Design review of the part shown in the three views and the two pictorial views. Dimensions are in mm from the part's minimum x, y and z. Round coordinates to 2 decimals unless told otherwise and drop trailing zeros. Order: outer loops, then holes, each group sorted by start corner. A loop starts at its lowest first (then second) coordinate and runs counter-clockwise, first axis right, second up.
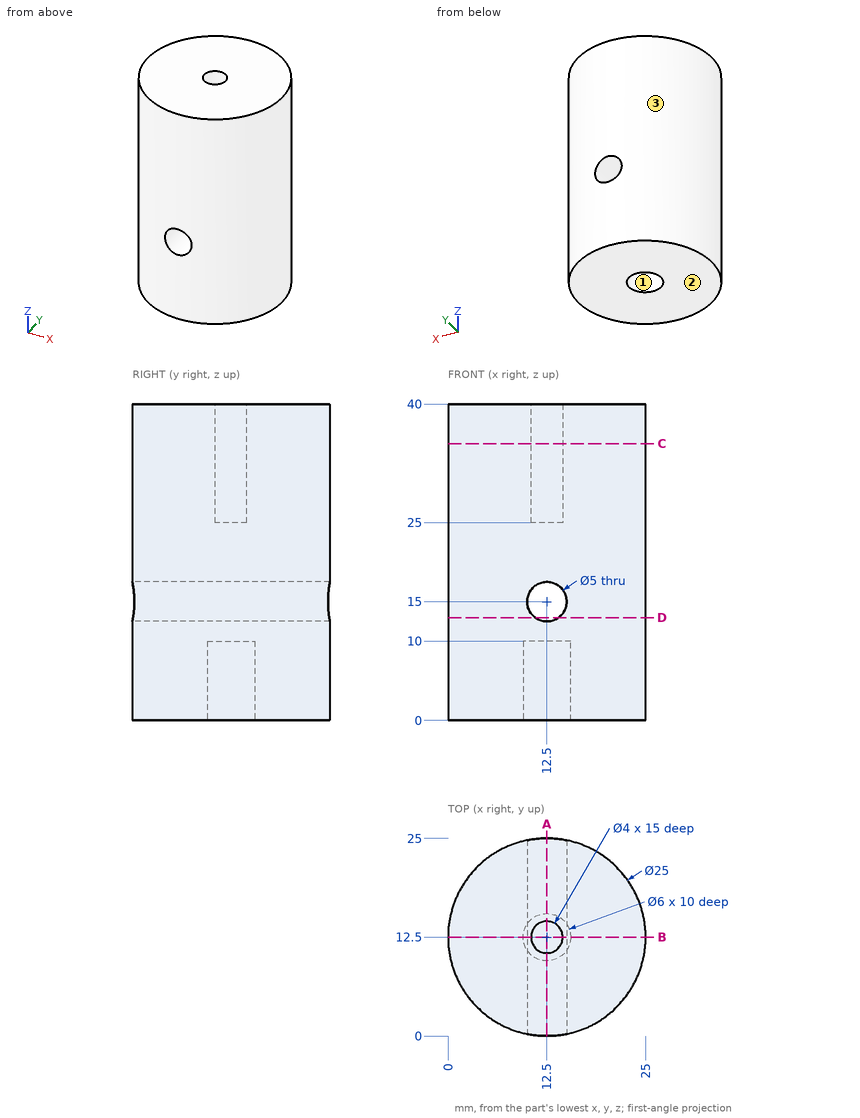
(1) Consider section B-B (y = 12.5). Write out the cut boundary in (x, z).
Data:
outline: (0, 0) - (9.5, 0) - (9.5, 10) - (15.5, 10) - (15.5, 0) - (25, 0) - (25, 40) - (14.5, 40) - (14.5, 25) - (10.5, 25) - (10.5, 40) - (0, 40) - close; hole circle Ø5 at (12.5, 15)
(2) Consider section A-A (x = 12.5). Write out the cut boundary in (y, z).
Data:
outline: (0, 0) - (9.5, 0) - (9.5, 10) - (15.5, 10) - (15.5, 0) - (25, 0) - (25, 12.5) - (0, 12.5) - close; (0, 17.5) - (25, 17.5) - (25, 40) - (14.5, 40) - (14.5, 25) - (10.5, 25) - (10.5, 40) - (0, 40) - close
(3) Consider section C-C (z = 35). Write out the cut boundary in (x, y).
Data:
outline: circle Ø25 at (12.5, 12.5); hole circle Ø4 at (12.5, 12.5)
(4) Consider section D-D (z = 13). Write out the cut boundary in (x, y).
Data:
outline: (11, 0.09) - (11, 24.91) arc R12.5 ccw to start; (14, 0.09) arc R12.5 ccw to (14, 24.91) - close
(5) Draft analysis for pull direction Y (two halves, no side actions). For the marked faces 1, 2 and 3, state which applies: pulls with the +Y half, pulls with the -Y half, needs draft (parallel to the pull), parting line crosses it, or undercut.
Data:
face 1: undercut
face 2: needs draft
face 3: parting line crosses it
(6) Insertion check: pin 1 (5 mm diameter, centred on x = 9, z = 31.5, fed in from -Y); pin 2 (1.2 mm diameter, centred on x = 13.5, y = 12.5, fed in from +Z); pin 3 (5 mm diameter, centred on x = 20, z = 19, fed in from +Y); pin 4 (3 mm diameter, centred on x = 12.5, z = 15, fed in from +Y). Each pin has a flat end and moves straight along its axis. Give the tip position at first contact, or say it passes through.
Data:
pin 1: stops at y = 0.04
pin 2: stops at z = 25
pin 3: stops at y = 23.96
pin 4: passes through
(7) To check wall thickness, follow probe 1 along Y at (x, z) = (12.5, 32); probe 2 along Y at (x, z) = (12.5, 6.75); probe 3 along Z at (x, y) = (12.5, 15). State the ranges of each line that lie inside material, in increasing order.
Data:
probe 1: y = 0 to 10.5, 14.5 to 25
probe 2: y = 0 to 9.5, 15.5 to 25
probe 3: z = 10 to 12.5, 17.5 to 40
